Design review of the part built by this model. Coordinates are the model's own, in mm. A direction names the side the tool comes from. Give positions to 0.01 mm unless a question says otherwise; leave off trailing zeros. Order: outer loops, then holes, each group sorted by start corner. A loop starts at its lowest first (then second) coordinate and runs counter-clockwise, first axis right, second up. Notation, with made-up numbers: M 15.25,84 L 52.25,84 A16 ccw 52.25,111 Z; hole C -26,1 d11. An arc over 180 degrees is marked long. Answer as a JSON object with one key per item and string values.
from build123d import *

# Parameters (mm, degrees)
F0_W     = 15
F0_H     = 60
F1_DEPTH = 5
F2_R     = 5
F3_R     = 7.5
F4_DEPTH = 30
F5_R     = 3
F6_DEPTH = 5
F7_R     = 7.5
F8_DEPTH = 5


with BuildPart() as f1:
    # F0 (on Top) → F1 (new body)
    with BuildSketch(Plane.XY):
        Rectangle(F0_W, F0_H)
    extrude(amount=F1_DEPTH)

    # F2
    f2_edges = [f1.edges().sort_by_distance(p)[0] for p in [
        (-7.5, 30, 2.5),
        (7.5, 30, 2.5),
        (7.5, -30, 2.5),
        (-7.5, -30, 2.5),
    ]]
    fillet(f2_edges, radius=F2_R)

    # F3 (on face) → F4 (join)
    with BuildSketch(Plane.XY.offset(5)):
        Circle(F3_R)
    extrude(amount=F4_DEPTH)

    # F5 (on face) → F6 (cut, through all)
    with BuildSketch(Plane(origin=(0, 0, 0), x_dir=(1, 0, 0), z_dir=(0, 0, -1))):
        with Locations((0, -25)):
            Circle(F5_R)
        with Locations((0, 25)):
            Circle(F5_R)
    extrude(amount=-F6_DEPTH, mode=Mode.SUBTRACT)

    # F7 (on Right) → F8 (join, symmetric)
    with BuildSketch(Plane.YZ):
        with Locations((0, 40)):
            Circle(F7_R)
    extrude(amount=F8_DEPTH, both=True)


solid = f1.part
(1) We need section C-C (z = 24.5). Write out the cut boundary in (x, y).
Checked values:
{"outline": "C 0,0 d15"}
(2) To check wall thickness, follow L1, parallel to Y at x = 0, z = 1.15; L2, parallel to X at y = -25, z = 2.85; L3, parallel to Z at x = 2.5, y = -12.5. State the ranges of each line that lie inside material, in increasing order. Write a range as from..to.
Checked values:
{"L1": "y = -30..-28, -22..22, 28..30", "L2": "x = -7.5..-3, 3..7.5", "L3": "z = 0..5"}
(3) Tool access review of faces 1 (the cylindrical face through (-7.493, 0.33, 19.79)), 2 (the flat face through (-5, 0, 41)), 3 (the cylindrical face through (-6.07, 28.5, 2.54)), 4 (the flat face through (6, 0, 35)), 5 (the cylindrical face through (6.07, 28.5, 2.54)): name each direction out of +Z, -Z, +X, -X, +Y, -Y from which nothing blocks a thin tool from reaching the whole face with its end or side.
Checked values:
{"face 1": "none", "face 2": "+Z, -X, +Y, -Y", "face 3": "+Z, -Z, -X, +Y", "face 4": "+Z, +X, +Y, -Y", "face 5": "+Z, -Z, +X, +Y"}
(4) We need section D-D (x = 6.75). Write out the cut boundary in (y, z).
Checked values:
{"outline": "M -27.63,0 L 27.63,0 L 27.63,5 L 3.27,5 L 3.27,35 L -3.27,35 L -3.27,5 L -27.63,5 Z"}
(5) Insertion check: pin 1 (7.5 mm diameter, centred on x = -1.5, y = -19, fed in from +Z); pin 2 (5 mm diameter, centred on x = -4, z = 8, fed in from +Y); pin 3 (0.6 mm diameter, centred on x = 0, y = 7, fed in from +Z). Each pin has a flat end and moves straight along its axis. Give the tip position at first contact, or say it passes through.
Checked values:
{"pin 1": "stops at z = 5", "pin 2": "stops at y = 7.35", "pin 3": "stops at z = 43.37"}
(6) We need section B-B (y = -6.5). Write out the cut boundary in (x, z), plus the area to 3 significant figures.
Checked values:
{"outline": "M -7.5,0 L 7.5,0 L 7.5,5 L 3.74,5 L 3.74,35 L -3.74,35 L -3.74,5 L -7.5,5 Z; M -5,36.26 L 5,36.26 L 5,43.74 L -5,43.74 Z", "area": "374 mm^2"}
(7) We need section A-A (x = 1.25). Write out the cut boundary in (y, z), plus the area to 3 significant figures.
Checked values:
{"outline": "M -30,0 L -27.73,0 L -27.73,5 L -30,5 Z; M -22.27,0 L 22.27,0 L 22.27,5 L 7.4,5 L 7.4,35 L 5.59,35 A7.5 ccw long -5.59,35 L -7.4,35 L -7.4,5 L -22.27,5 Z; M 27.73,0 L 30,0 L 30,5 L 27.73,5 Z", "area": "847 mm^2"}
(8) Draft analysis for pull direction X (two halves, no side actions). For faces 6 (the cylindrical face through (-0.65, -22.07, 2.46)), 7 (the flat face through (0, -30, 2)), 8 (the flat face through (5, 0, 41)), state which applies: +X half, -X half, draft (parallel to the pull), parting line (faces both ways), or undercut.
Checked values:
{"face 6": "undercut", "face 7": "draft", "face 8": "+X half"}
